Source: CAD feature listing. Evaluate the final solid. Frame: model axes, mm. A direction names the side the tool comes from. Round coordinates to 2 decimals unless told otherwise and drop trailing zeros. Order: outer loops, then holes, each group sorted by start corner. A loop starts at its lowest first (then second) coordinate and runs counter-clockwise, first axis right, second up. Notation, with made-up numbers: (10, 7) - (64, 7) arc R10 ccw to (64, 21) - close; hole circle Ø4 at (84, 7). An arc over 180 degrees is marked (long way). Use one line per item in the form item = value. Start each with the question number.
Q1. Pin query (flat end, axial travel): pin 1 Ø0.9 at (x, z) = (-7, 7) entering from -Y. Return the tip coordinate at first contact, or that it passes through.
Q2. Cut plane A-A, the plane y = 1.8. Return the cut outline in (x, z), and give its area (3 significant figures).
Q3. Cut plane C-C, the plane z = 4.5. Return the cut outline in (x, y), and give its area (3 significant figures).
Q4. Draft query along X for faces 1 (the flat face through (0, 3, 0)), 2 (the flat face through (8, 1, 0)), 3 (the flat face through (3, 2, 0)). Return one class per face: released by +X, released by -X, zero draft, split by the parting line, or undercut.
Q5. Cut plane D-D, the plane x = 3. Return the cut outline in (y, z), and give its area (3 significant figures).
Q6. Ray query, line 1 (Z direction, x = 7, y = 0.5); line 2 (Z direction, x = -3.5, y = 1.5); line 3 (X direction, y = 0.9, z = 1.5). Return the intervals inside material, ascending. Write a range as [from, to].
Q7. Set-up query: faces 4 (the flat face through (0, 0, 6.5)), 5 (the cylindrical face through (-7.75, 0.99, 7.03)). Return all of +Z, -Z, +X, -X, +Y, -Y with unobstructed straight access to the full face (end or side cutting, diameter ignored); none if empty.
Q8. Cut plane B-B, the plane x = 0. Return the cut outline in (y, z), and give its area (3 significant figures).
from build123d import *

# Parameters (mm, degrees)
SKETCH1_W           = 16
SKETCH1_H           = 16
BOSS_EXTRUDE1_DEPTH = 3
SKETCH2_W           = 12
SKETCH2_H           = 12
SKETCH2_R           = 2.5
CUT_EXTRUDE1_DEPTH  = 2
SKETCH3_R           = 0.75
CUT_EXTRUDE2_DEPTH  = 2


with BuildPart() as part:
    # Sketch1 → Boss-Extrude1 (new body)
    with BuildSketch(Plane(origin=(0, 0, 0), x_dir=(1, 0, 0), z_dir=(0, 1, 0))):
        Rectangle(SKETCH1_W, SKETCH1_H)
    extrude(amount=BOSS_EXTRUDE1_DEPTH)

    # Sketch2 → Cut-Extrude1 (cut)
    with BuildSketch(Plane.XZ):
        Rectangle(SKETCH2_W, SKETCH2_H)
        Circle(SKETCH2_R, mode=Mode.SUBTRACT)
    extrude(amount=-CUT_EXTRUDE1_DEPTH, mode=Mode.SUBTRACT)

    # Sketch3 → Cut-Extrude2 (cut)
    with BuildSketch(Plane.XZ):
        with Locations((-7, 7)):
            Circle(SKETCH3_R)
        with Locations((7, 7)):
            Circle(SKETCH3_R)
        with Locations((7, -7)):
            Circle(SKETCH3_R)
        with Locations((-7, -7)):
            Circle(SKETCH3_R)
    extrude(amount=-CUT_EXTRUDE2_DEPTH, mode=Mode.SUBTRACT)


solid = part.part
Completed:
q1.pin_1 = 2
q2.outline = (-8, -8) - (8, -8) - (8, 8) - (-8, 8) - close; circle Ø5 at (0, 0); hole circle Ø1.5 at (-7, -7); hole circle Ø1.5 at (-7, 7); hole (-6, -6) - (6, -6) - (6, 6) - (-6, 6) - close; hole circle Ø1.5 at (7, -7); hole circle Ø1.5 at (7, 7)
q2.area = 125 mm2
q3.outline = (-8, 0) - (-6, 0) - (-6, 2) - (6, 2) - (6, 0) - (8, 0) - (8, 3) - (-8, 3) - close
q3.area = 24.0 mm2
q4.face_1 = zero draft
q4.face_2 = released by +X
q4.face_3 = undercut
q5.outline = (0, -8) - (3, -8) - (3, 8) - (0, 8) - (0, 6) - (2, 6) - (2, -6) - (0, -6) - close
q5.area = 24.0 mm2
q6.line_1 = [-8, -7.75], [-6.25, 6.25], [7.75, 8]
q6.line_2 = [-8, -6], [6, 8]
q6.line_3 = [-8, -6], [-2, 2], [6, 8]
q7.face_4 = +Z, -Z, +X, -X, -Y
q7.face_5 = -Y
q8.outline = (0, -8) - (3, -8) - (3, 8) - (0, 8) - (0, 6) - (2, 6) - (2, 2.5) - (0, 2.5) - (0, -2.5) - (2, -2.5) - (2, -6) - (0, -6) - close
q8.area = 34.0 mm2
